```python
from build123d import *

# Parameters (mm, degrees)
BOSS_EXTRUDE1_DEPTH                            = 4.9
SKETCH2_W                                      = 4.75
SKETCH2_H                                      = 83.9
BOSS_EXTRUDE2_DEPTH                            = 22.9
CUT_EXTRUDE1_START                             = -4.75
CUT_EXTRUDE1_DEPTH                             = 4.75
CSK_FOR_M6_FLAT_HEAD_MACHINE_SCREW1_AT_2_COUNT = 2
CSK_FOR_M6_FLAT_HEAD_MACHINE_SCREW1_AT_2_PITCH = 59.791303716
SKETCH8_W                                      = 41.834673512
SKETCH8_H                                      = 83.9
CUT_REVOLVE4_ANGLE                             = 3


# Read off the part's stored shape, not the designer's step: Cut-Extrude1
with BuildPart() as part:
    # Sketch1 → Boss-Extrude1 (new body)
    with BuildSketch(Plane.XY):
        with BuildLine():
            Line((-17.45, -41.95), (22.45, -41.95))
            Line((22.45, -41.95), (22.45, 41.95))
            Line((22.45, 41.95), (-17.45, 41.95))
            ThreePointArc((-17.45, 41.95), (-20.985533906, 40.485533906), (-22.45, 36.95))
            Line((-22.45, 36.95), (-22.45, -36.95))
            ThreePointArc((-22.45, -36.95), (-20.985533906, -40.485533906), (-17.45, -41.95))
        make_face()
    extrude(amount=BOSS_EXTRUDE1_DEPTH)

    # Sketch2 → Boss-Extrude2 (add)
    with BuildSketch(Plane.XY.offset(4.9)):
        with Locations((20.075, 0)):
            Rectangle(SKETCH2_W, SKETCH2_H)
    extrude(amount=BOSS_EXTRUDE2_DEPTH)

    # Cut-Extrude1 outline → Cut-Extrude1 (cut)
    with BuildSketch(Plane(origin=(22.45, 0, 0), x_dir=(0, 0, -1), z_dir=(1, 0, 0)).offset(CUT_EXTRUDE1_START)):
        with BuildLine():
            Line((-27.8, 41.95), (-27.800002133, 36.67650399))
            ThreePointArc((-27.800002133, 36.67650399), (-26.255432728, 40.405429091), (-22.526508249, 41.95))
            Line((-22.526508249, 41.95), (-27.8, 41.95))
        make_face()
        with BuildLine():
            Line((-27.8, -36.676506119), (-27.8, -41.95))
            Line((-27.8, -41.95), (-22.526505934, -41.95))
            ThreePointArc((-22.526505934, -41.95), (-26.255429337, -40.405429468), (-27.8, -36.676506119))
        make_face()
    extrude(amount=CUT_EXTRUDE1_DEPTH, mode=Mode.SUBTRACT)

    # Sketch6 → CSK for M6 Flat Head Machine Screw1 (revolve, cut)
    with BuildSketch(Plane(origin=(2.5, 29.895651858, 0), x_dir=(0, 1, 0), z_dir=(1, 0, 0))):
        Polygon((0, 0), (0, 4.9), (3.3, 4.9), (3.3, 3), (6.3, 0), align=None)
    csk_for_m6_flat_head_machine_screw1 = revolve(axis=Axis((2.5, 29.895651858, -6.35), (0, 0, 1)), mode=Mode.SUBTRACT)

    # CSK for M6 Flat Head Machine Screw1 at 2: CSK for M6 Flat Head Machine Screw1 ×2
    with Locations(*[(0, -i * CSK_FOR_M6_FLAT_HEAD_MACHINE_SCREW1_AT_2_PITCH, 0) for i in range(1, CSK_FOR_M6_FLAT_HEAD_MACHINE_SCREW1_AT_2_COUNT)]):
        add(csk_for_m6_flat_head_machine_screw1, mode=Mode.SUBTRACT)

    # Sketch8 → Cut-Revolve4 (revolve, cut)
    with BuildSketch(Plane(origin=(22.45, 0, 0), x_dir=(0, 0, -1), z_dir=(1, 0, 0))):
        with Locations((-20.917336756, 0)):
            Rectangle(SKETCH8_W, SKETCH8_H)
    revolve(axis=Axis((22.45, -41.95, 0), (0, -1, 0)), revolution_arc=CUT_REVOLVE4_ANGLE, mode=Mode.SUBTRACT)


solid = part.part
```
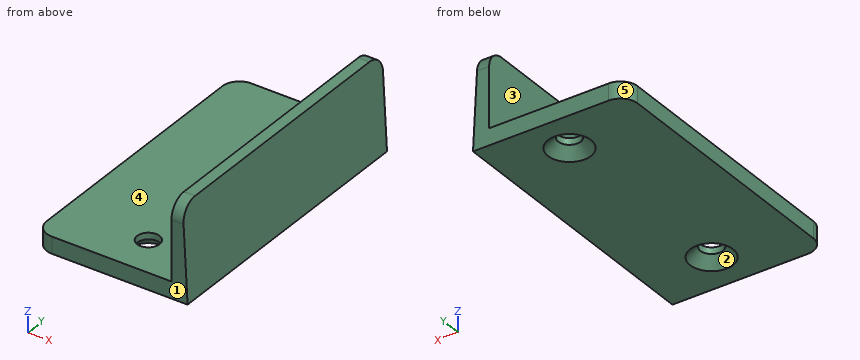
Verification items for the finished model (mm, model axes). Face numbers are marked on the shaded views. A direction names the side the tool comes from. Coordinates: 2 decimals unless noted, no trailing zeros. Write each loop counter-clockwise with the first axis right and the second up, starting at its lowest first coordinate (ties: lowest second). Pieces come first, ordered by that corner, then holes. Notation, with made-up numbers: M 53,68 L 59,68 A13 ccw 59,88 Z; hole C 87,46 d4. An arc over 180 degrees is marked long. Answer as a JSON object with one key per item and string values. Group by question number.
(1) Tool access check on the marked faces 4 and 5. Record the directions out of +Z, -Z, +X, -X, +Y, -Y that give a thin tool (end or side, any length) a straight path to the whole face; none if there is none.
(2) Cross-section at B-B, the plane y = -12. Record the cut outline in (x, z).
(3) Gauge pin test, flat ends, axial feed: pin 1 (3 mm diameter, centred on x = 7, y = 14.5, fed in from +Z); pin 2 (7 mm diameter, centred on y = 7, z = 21.5, fed in from -X); pin 3 (10.5 mm diameter, centred on x = 2.5, y = 29.9, fed in from -Z); pin 4 (4 mm diameter, centred on x = 2.5, y = -29.9, fed in from -Z). Record the tip position at first contact, or that the pin passes through.
(4) Material ranges on line 1 (Y direction, x = 2.5, z = 3.45); line 2 (Z direction, x = -11, y = -9.5); line 3 (Z direction, x = 20, y = -37), recorded low to high.
(5) Release check for a two-part mould opening along Y. For the marked faces 1, 2 and 3 record: +Y half, -Y half, draft (parallel to the pull), parting line (faces both ways), or undercut.
(6) Cross-section at C-C, the plane x = -7. Record the cut outline in (y, z), and give its area (3 significant figures).
(7) Cross-section at D-D, the plane z = 15.25. Record the cut outline in (x, y), and give its area (3 significant figures).
(8) Cross-section at A-A, the plane x = 2.5. Record the cut outline in (y, z), and give its area (3 significant figures).
Reply:
{
 "1": {"face 4": "+Z, -X, +Y, -Y", "face 5": "+Z, -Z, -X, +Y"},
 "2": {"outline": "M -22.45,0 L 22.45,0 L 20.99,27.8 L 17.7,27.8 L 17.7,4.9 L -22.45,4.9 Z"},
 "3": {"pin 1": "z = 4.9", "pin 2": "x = 17.7", "pin 3": "z = 1.05", "pin 4": "through"},
 "4": {"line 1": "-41.95 to -33.2, -26.6 to 26.6, 33.2 to 41.95", "line 2": "0 to 4.9", "line 3": "0 to 27.79"},
 "5": {"face 1": "-Y half", "face 2": "undercut", "face 3": "draft"},
 "6": {"outline": "M -41.95,0 L 41.95,0 L 41.95,4.9 L -41.95,4.9 Z", "area": "411 mm²"},
 "7": {"outline": "M 17.7,-41.95 L 21.65,-41.95 L 21.65,41.95 L 17.7,41.95 Z", "area": "331 mm²"},
 "8": {"outline": "M -41.95,0 L -36.2,0 L -33.2,3 L -33.2,4.9 L -41.95,4.9 Z; M -26.6,3 L -23.6,0 L 23.6,0 L 26.6,3 L 26.6,4.9 L -26.6,4.9 Z; M 33.2,3 L 36.2,0 L 41.95,0 L 41.95,4.9 L 33.2,4.9 Z", "area": "328 mm²"}
}
